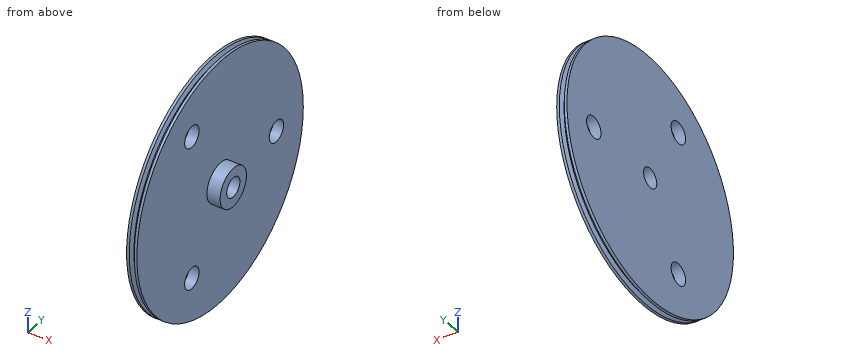
from build123d import *

# Parameters (mm, degrees)
SKETCH3_R          = 19.05
CUT_EXTRUDE1_DEPTH = 344.324834049
SKETCH4_R          = 20.893502845
CUT_EXTRUDE2_DEPTH = 344.324834049


with BuildPart() as part:
    # Sketch2 → Revolve1 (revolve)
    with BuildSketch(Plane.XY):
        Polygon((0, 0), (0, 240.665), (5.08, 240.665), (8.781317037, 232.7275), (10.903682963, 232.7275), (14.605, 240.665), (19.685, 240.665), (19.685, 38.1), (45.085, 38.1), (45.085, 0), align=None)
    revolve(axis=Axis((45.085, 0, 0), (-1, 0, 0)))

    # Sketch3 → Cut-Extrude1 (cut, through all)
    with BuildSketch(Plane(origin=(45.085, 0, 0), x_dir=(0, 0, -1), z_dir=(1, 0, 0))):
        with Locations(Location((0, 0, 0), (0, 0, 90))):
            Circle(SKETCH3_R)
    extrude(amount=-CUT_EXTRUDE1_DEPTH, mode=Mode.SUBTRACT)

    # Sketch4 → Cut-Extrude2 (cut, through all)
    with BuildSketch(Plane.ZY):
        with Locations(Location((0, 163.022805962, 0), (0, 0, 270))):
            Circle(SKETCH4_R)
        with Locations(Location((141.181891359, -81.511402981, 0), (0, 0, 270))):
            Circle(SKETCH4_R)
        with Locations(Location((-141.181891359, -81.511402981, 0), (0, 0, 270))):
            Circle(SKETCH4_R)
    extrude(amount=-CUT_EXTRUDE2_DEPTH, mode=Mode.SUBTRACT)


solid = part.part
Build history of the part. All positions in model axes, mm. Coordinates: 2 decimals unless noted, no trailing zeros. Write each loop counter-clockwise with the first axis right and the second up, starting at its lowest first coordinate (ties: lowest second). Pieces come first, ordered by that corner, then holes. Notation, with made-up numbers: (-39, 17) -> (-3, 17) arc R19 ccw to (-3, 50) -> close; hole circle Ø5 at (80, 82). An arc over 180 degrees is marked (long way). Use CSV: the item, a comma, the result in double quotes. Start each with the question number.
Q1. Flat gauge pins, fed straight in: pin 1 Ø1 at (x, y) = (29, -5) entering from +Z; pin 2 Ø3 at (y, z) = (-60.5, 169) entering from +X (3 decimals); pin 3 Ø8 at (x, z) = (25.5, -5) entering from +Y; pin 4 Ø6 at (y, z) = (-41, 9) entering from -X. Where does each tip first touch, or does it go through?
Q2. Cut at A-A, the plane z = 0. State how many separate pieces and enclosed holes the cut face has, then the cut area to 3 significant figures.
Q3. Cut at C-C, the plane x = 25.5. List the corners of the cut face in (y, z).
Q4. Drill centre lines: probe 1 along Z at (x, y) = (33.5, 0); probe 2 along X at (y, z) = (-93.5, -26) (3 decimals); probe 3 along Y at (x, z) = (35, 21). Where is each one in solid material? Low to high.
Checked values:
1,pin 1,"stops at z = 37.83"
1,pin 2,"stops at x = 19.685"
1,pin 3,"stops at y = 38.09"
1,pin 4,"stops at x = 0"
2,separate pieces,"3"
2,enclosed holes,"0"
2,area,"8,780 mm²"
3,outline,"circle Ø76.2 at (0, 0); hole circle Ø38.1 at (0, 0)"
4,probe 1,"z = -38.1 to -19.05, 19.05 to 38.1"
4,probe 2,"x = 0 to 19.685"
4,probe 3,"y = -31.79 to 31.79"
